Could you check a few things on this model? Use its own coordinates, in mm. Face numbers are marked on the shaded views. A direction names the side the tool comes from. Give positions to 0.01 mm unless a question says otherwise; leave off trailing zeros. Loops run counter-clockwise (first coordinate to the right, second up) from the corner with the lowest first, then second, coordinate; pieces in that order, holes last. Notation, with made-up numbers: (56.25, 73.5) -> (80.25, 73.5) arc R21 cw to (80.25, 88.5) -> close; hole circle Ø7 at (87, -2.75). An arc over 180 degrees is marked (long way). Write item = value, one per line. Start each with the question number.
1) I want a section at C-C (y = 0). List the corners of the cut face in (x, z) for me.
2) If we mould it in two halves opening along X, with no side actions, what happens to the marked faces 3, 4 and 5? For each: +X half, -X half, draft (parallel to the pull), parting line (faces both ways), or undercut.
3) I want a section at D-D (x = 0). List the corners of the cut face in (y, z) for me.
4) On a 3-axis mill with a long thin cutter (end or side, diameter ignored), from which of +Z, -Z, +X, -X, +Y, -Y can I reach the whole of each face in a straight line? I mean the marked faces 1 and 2. Say none if no direction works.
5) I want a section at B-B (z = 2.5). List the corners of the cut face in (x, y) for me.
6) I want a section at A-A (y = 4.75). List the corners of the cut face in (x, z) for me.
7) I need wall thicknesses on probe 1 along Z at (x, y) = (0, 24.5); probe 2 along Y at (x, z) = (-3.5, 2.45); probe 3 along X at (y, z) = (6.25, 3.15). Which ranges of each line are inside material? Lowest first, please. Write a range as from..to.
8) I'm going to push a flat-ended pin straight in: pin 1 Ø2.5 at (x, z) = (4, 2.5) entering from -Y. Where does the tip first touch, or does it pass through?
from build123d import *

# Parameters (mm, degrees)
BOSS_EXTRUDE1_DEPTH             = 5
F_29_0_136_DIAMETER_HOLE1_D     = 3.4544
F_29_0_136_DIAMETER_HOLE1_DEPTH = 4
CIRPATTERN1_START               = -30
CIRPATTERN1_OUTLINE_R           = 1.7272
CIRPATTERN1_DEPTH               = 4
CIRPATTERN1_START_2             = 22
CIRPATTERN1_2_OUTLINE_R         = 1.7272
CIRPATTERN1_2_DEPTH             = 4


# Read off the part's stored shape, not the designer's step: CirPattern1
with BuildPart() as part:
    # Sketch1 → Boss-Extrude1 (new body)
    with BuildSketch(Plane.XY):
        Polygon((-30, -2.5), (-26, -2.5), (-26, 6.769552622), (-10.769552622, 22), (10.769552622, 22), (26, 6.769552622), (26, -2.5), (30, -2.5), (30, 9.840620434), (13.840620434, 26), (-13.840620434, 26), (-30, 9.840620434), align=None)
    extrude(amount=BOSS_EXTRUDE1_DEPTH)

    # #29 (0.136) Diameter Hole1
    with Locations(Plane(origin=(30, 0, 0), x_dir=(0, 0, -1), z_dir=(1, 0, 0))):
        with Locations((-2.5, 0)):
            Hole(F_29_0_136_DIAMETER_HOLE1_D / 2, depth=F_29_0_136_DIAMETER_HOLE1_DEPTH)

    # CirPattern1 outline → CirPattern1 (cut)
    with BuildSketch(Plane.YZ.offset(CIRPATTERN1_START)):
        with Locations((0, 2.5)):
            Circle(CIRPATTERN1_OUTLINE_R)
    extrude(amount=CIRPATTERN1_DEPTH, mode=Mode.SUBTRACT)

    # CirPattern1 2 outline → CirPattern1 2 (cut)
    with BuildSketch(Plane(origin=(0, 0, 0), x_dir=(1, 0, 0), z_dir=(0, 1, 0)).offset(CIRPATTERN1_START_2)):
        with Locations((0, -2.5)):
            Circle(CIRPATTERN1_2_OUTLINE_R)
    extrude(amount=CIRPATTERN1_2_DEPTH, mode=Mode.SUBTRACT)


solid = part.part
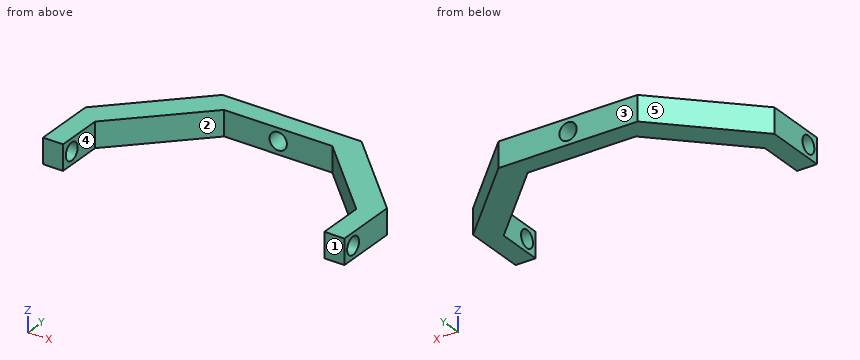
Answer list:
q1.outline = (-30, 0) -> (-26, 0) -> (-26, 0.77) -> (-30, 0.77) -> close; (-30, 4.23) -> (-26, 4.23) -> (-26, 5) -> (-30, 5) -> close; (26, 0) -> (30, 0) -> (30, 0.77) -> (26, 0.77) -> close; (26, 4.23) -> (30, 4.23) -> (30, 5) -> (26, 5) -> close
q2.face_3 = draft
q2.face_4 = undercut
q2.face_5 = -X half
q3.outline = (22, 0) -> (26, 0) -> (26, 0.77) -> (22, 0.77) -> close; (22, 4.23) -> (26, 4.23) -> (26, 5) -> (22, 5) -> close
q4.face_1 = +Z, -Z, +X, -X, -Y
q4.face_2 = +Z, -Z, -Y
q5.outline = (-30, -2.5) -> (-26, -2.5) -> (-26, -1.73) -> (-30, -1.73) -> close; (-30, 1.73) -> (-26, 1.73) -> (-26, 6.77) -> (-10.77, 22) -> (-1.73, 22) -> (-1.73, 26) -> (-13.84, 26) -> (-30, 9.84) -> close; (1.73, 22) -> (10.77, 22) -> (26, 6.77) -> (26, 1.73) -> (30, 1.73) -> (30, 9.84) -> (13.84, 26) -> (1.73, 26) -> close; (26, -2.5) -> (30, -2.5) -> (30, -1.73) -> (26, -1.73) -> close
q6.outline = (-30, 0) -> (-26, 0) -> (-26, 5) -> (-30, 5) -> close; (26, 0) -> (30, 0) -> (30, 5) -> (26, 5) -> close
q7.probe_1 = 0..0.77, 4.23..5
q7.probe_2 = 22..26
q7.probe_3 = -30..-26, 26..30
q8.pin_1 = 22
